Build history of the part. All positions in model axes, mm. A direction names the side the tool comes from. Round coordinates to 2 decimals unless told otherwise and drop trailing zeros. Write each loop counter-clockwise with the first axis right and the second up, starting at its lowest first coordinate (ties: lowest second). Pieces come first, ordered by that corner, then holes. Notation, with made-up numbers: (35, -25) -> (77, -25) arc R6 cw to (77, -19) -> close; hole circle Ø11 at (46.5, 48). An arc over 180 degrees is marked (long way). Return JSON: item names as keys, results as strings.
from build123d import *

# Parameters (mm, degrees)
F1_DEPTH    = 60
F2_R        = 5
F3_DEPTH    = 25
F4_R        = 2
F5_DEPTH    = 25
F6_SIZE     = 2
F7_SIZE     = 2
F8_R        = 2.5
F9_T1_DEPTH = 71.4564392374


# Not quite as in the source:
# - a fillet or chamfer that OpenCascade refuses, or shapes differently, is made with other operations: its cross-section is extruded or revolved along the edge and cut away or added


with BuildPart() as f1:
    # F0 (on Top) → F1 (new body)
    with BuildSketch(Plane.XY):
        with BuildLine():
            Line((0, 4), (0, 0))
            Line((0, 0), (30.5437369547, 0))
            ThreePointArc((30.5437369547, 0), (38.4878384458, 4.7701948627), (38.0108483544, 14.0241663334))
            Line((38.0108483544, 14.0241663334), (18.0912535296, 43.6294428556))
            Line((18.0912535296, 43.6294428556), (14.7725373519, 41.3964800408))
            Line((14.7725373519, 41.3964800408), (33.0393692072, 14.2476041216))
            Line((33.0393692072, 14.2476041216), (34.6921321767, 11.7912035185))
            ThreePointArc((34.6921321767, 11.7912035185), (34.957126672, 6.650108257), (30.5437369547, 4))
            Line((30.5437369547, 4), (0, 4))
        make_face()
    extrude(amount=F1_DEPTH)

    # F2 (on face) → F3 (cut)
    with BuildSketch(Plane(origin=(32.6608671723, 21.9755164324, 0), x_dir=(-0.5582407037, 0.8296790444, 0), z_dir=(0.8296790444, 0.5582407037, 0))):
        with Locations((6.0991603551, 44)):
            Circle(F2_R)
        with Locations((6.0991603551, 16)):
            Circle(F2_R)
    extrude(amount=-F3_DEPTH, mode=Mode.SUBTRACT)

    # F4 (on face) → F5 (cut)
    with BuildSketch(Plane.XZ):
        with Locations((12, 12.7154784277)):
            Circle(F4_R)
        with Locations((12, 50)):
            Circle(F4_R)
    extrude(amount=-F5_DEPTH, mode=Mode.SUBTRACT)

    # F6
    f6_edges = [f1.edges().sort_by_distance(p)[0] for p in [
        (10, 4, 12.715478),
    ]]
    chamfer(f6_edges, length=F6_SIZE)

    # F7
    f7_edges = [f1.edges().sort_by_distance(p)[0] for p in [
        (10, 4, 50),
    ]]
    chamfer(f7_edges, length=F7_SIZE)

    # F8
    f8_edges = [f1.edges().sort_by_distance(p)[0] for p in [
        (18.091254, 43.629443, 30),
    ]]
    fillet(f8_edges, radius=F8_R)

    # F9: fillet of radius 2.5 on 1 edges, made by hand

    # F9_s2 → F9_t1 (cut)
    with BuildSketch(Plane.XY.offset(-5.7282196187)):
        with BuildLine():
            ThreePointArc((16.0170559185, 42.2338410964), (15.6260243102, 40.8594889036), (16.0516274923, 39.495446529))
            Line((16.0516274923, 39.495446529), (14.7725373519, 41.3964800408))
            Line((14.7725373519, 41.3964800408), (16.0170559185, 42.2338410964))
        make_face()
    extrude(amount=F9_T1_DEPTH, mode=Mode.SUBTRACT)


solid = f1.part
Q1. Two-plate mould, pull along Z, no slides. Class faces 1 (the cylindrical face through (26.119, 28.165, 48.216)), 2 (the flat face through (30, 20, 60)), 3 (the cylindrical face through (10.41, 0.99, 11.5)), 4 (the cylindrical face through (38.423, 4.65, 29.58)): +Z half, -Z half, draft (parallel to the pull), parting line (faces both ways), or undercut.
Verdict:
{"face 1": "undercut", "face 2": "+Z half", "face 3": "undercut", "face 4": "draft"}
Q2. Wall check: L1, parallel to Z at x = 12, y = 0.9; L2, parallel to Y at x = 3.5, z = 40; L3, parallel to Y at x = 16.5, z = 33. Give the ranges that are in metal, low to high.
Verdict:
{"L1": "z = 0 to 10.72, 14.72 to 48, 52 to 60", "L2": "y = 0 to 4", "L3": "y = 0 to 4, 38.83 to 42.49"}
Q3. Saw through at C-C on x = 17. List the corners of the cut face in (y, z).
Verdict:
{"outline": "(0, 0) -> (4, 0) -> (4, 60) -> (0, 60) -> close; (38.09, 0) -> (42.63, 0) -> (42.63, 60) -> (38.09, 60) -> close"}
Q4. Saw through at A-A on x = 12. List the corners of the cut face in (y, z), then the cut area to 3 significant figures.
Verdict:
{"outline": "(0, 0) -> (4, 0) -> (4, 8.72) -> (2, 10.72) -> (0, 10.72) -> close; (0, 14.72) -> (2, 14.72) -> (4, 16.72) -> (4, 46) -> (2, 48) -> (0, 48) -> close; (0, 52) -> (2, 52) -> (4, 54) -> (4, 60) -> (0, 60) -> close", "area": "200 mm²"}
Q5. Saw through at D-D on z = 8. List the corners of the cut face in (x, y), then the cut area to 3 significant figures.
Verdict:
{"outline": "(0, 0) -> (30.54, 0) arc R9 ccw to (38.01, 14.02) -> (19.49, 41.56) arc R2.5 ccw to (16.02, 42.23) arc R2.5 ccw to (16.05, 39.5) -> (34.69, 11.79) arc R5 cw to (30.54, 4) -> (0, 4) -> close", "area": "323 mm²"}
Q6. Saw through at B-B on z = 50. List the corners of the cut face in (x, y).
Verdict:
{"outline": "(0, 0) -> (10, 0) -> (10, 2) -> (8, 4) -> (0, 4) -> close; (14, 0) -> (30.54, 0) arc R9 ccw to (38.01, 14.02) -> (19.49, 41.56) arc R2.5 ccw to (16.02, 42.23) arc R2.5 ccw to (16.05, 39.5) -> (34.69, 11.79) arc R5 cw to (30.54, 4) -> (16, 4) -> (14, 2) -> close"}
Q7. 3-axis set-ups, long thin cutter, end or side, ignore diameter. For faces 5 (the flat face through (0, 2, 30)), 6 (the flat face through (15, 4, 30)): which of +Z, -Z, +X, -X, +Y, -Y reach the whole face in a straight line?
Verdict:
{"face 5": "+Z, -Z, -X, +Y, -Y", "face 6": "+Z, -Z, -X"}
Q8. Pin check, flat tips, straight feed: pin 1 Ø1.5 at (y, z) = (24, 26) entering from -X; pin 2 Ø9 at (x, z) = (9.5, 43) entering from +Y; pin 3 Ø6.5 at (x, z) = (12, 12.72) entering from +Y. Stop position of each tip, or through.
Verdict:
{"pin 1": "stops at x = 25.97", "pin 2": "stops at y = 4", "pin 3": "stops at y = 3.25"}
